```python
from build123d import *

# Parameters (mm, degrees)
SKETCH1_W               = 21.59
SKETCH1_H               = 46.99
BOSS_EXTRUDE1_DEPTH     = 76.2
SKETCH2_R               = 14.605
CUT_EXTRUDE1_DEPTH      = 93.090326311
CUT_EXTRUDE2_DEPTH      = 93.090326311
CUT_EXTRUDE3_REACH      = 94.09
SKETCH4_R               = 2.54
CUT_EXTRUDE4_REACH      = 94.09
CUT_EXTRUDE4_END_RADIUS = 14.605
SKETCH5_R               = 2.54
CHAMFER1_SIZE           = 2.54


with BuildPart() as part:
    # Sketch1 → Boss-Extrude1 (new body)
    with BuildSketch(Plane.XY):
        with Locations((10.795, 23.495)):
            Rectangle(SKETCH1_W, SKETCH1_H)
    extrude(amount=BOSS_EXTRUDE1_DEPTH)

    # Sketch2 → Cut-Extrude1 (cut, through all)
    with BuildSketch(Plane(origin=(21.59, 0, 0), x_dir=(0, 0, -1), z_dir=(1, 0, 0))):
        with Locations((-38.1, 23.495)):
            Circle(SKETCH2_R)
    extrude(amount=-CUT_EXTRUDE1_DEPTH, mode=Mode.SUBTRACT)

    # Sketch3 → Cut-Extrude2 (cut, through all)
    with BuildSketch(Plane(origin=(21.59, 0, 0), x_dir=(0, 0, -1), z_dir=(1, 0, 0))):
        Polygon((-50.8, 0), (-76.2, 23.495), (-76.2, 0), align=None)
    extrude(amount=-CUT_EXTRUDE2_DEPTH, mode=Mode.SUBTRACT)

    # Sketch4 → Cut-Extrude3 (cut, up to next)
    with BuildSketch(Plane(origin=(0, 46.99, 0), x_dir=(1, 0, 0), z_dir=(0, 1, 0)), mode=Mode.PRIVATE) as cut_extrude3_sk1:
        with Locations(Location((10.795, -12.7, 0), (0, 0, 270))):
            Circle(SKETCH4_R)
    cut_extrude3_tool1 = extrude(cut_extrude3_sk1.sketch, amount=-CUT_EXTRUDE3_REACH, mode=Mode.PRIVATE) & part.part
    # Sketch4 → Cut-Extrude3 (cut, up to next)
    with BuildSketch(Plane(origin=(0, 46.99, 0), x_dir=(1, 0, 0), z_dir=(0, 1, 0)), mode=Mode.PRIVATE) as cut_extrude3_sk2:
        with Locations(Location((10.795, -38.1, 0), (0, 0, 270))):
            Circle(SKETCH4_R)
    cut_extrude3_tool2 = extrude(cut_extrude3_sk2.sketch, amount=-CUT_EXTRUDE3_REACH, mode=Mode.PRIVATE) & part.part
    # Sketch4 → Cut-Extrude3 (cut, up to next)
    with BuildSketch(Plane(origin=(0, 46.99, 0), x_dir=(1, 0, 0), z_dir=(0, 1, 0)), mode=Mode.PRIVATE) as cut_extrude3_sk3:
        with Locations(Location((10.795, -63.5, 0), (0, 0, 270))):
            Circle(SKETCH4_R)
    cut_extrude3_tool3 = extrude(cut_extrude3_sk3.sketch, amount=-CUT_EXTRUDE3_REACH, mode=Mode.PRIVATE) & part.part
    add(cut_extrude3_tool1.solids().sort_by_distance((10.795, 46.99, 12.7))[0], mode=Mode.SUBTRACT)
    add(cut_extrude3_tool2.solids().sort_by_distance((10.795, 46.99, 38.1))[0], mode=Mode.SUBTRACT)
    add(cut_extrude3_tool3.solids().sort_by_distance((10.795, 46.99, 63.5))[0], mode=Mode.SUBTRACT)

    # Cut-Extrude4: up to this cylinder (the profile starts outside it)
    cut_extrude4_end = Plane(origin=(10.795, 23.495, 38.1), z_dir=(1, 0, 0)) * Cylinder(CUT_EXTRUDE4_END_RADIUS, 218.39, mode=Mode.PRIVATE)
    # Sketch5 → Cut-Extrude4 (cut, up to the surface)
    with BuildSketch(Plane.XZ, mode=Mode.PRIVATE) as cut_extrude4_sk1:
        with Locations(Location((10.795, 39.6875, 0), (0, 0, 270))):
            Circle(SKETCH5_R)
    cut_extrude4_tool1 = extrude(cut_extrude4_sk1.sketch, amount=-CUT_EXTRUDE4_REACH, mode=Mode.PRIVATE) - cut_extrude4_end
    add(cut_extrude4_tool1.solids().sort_by_distance((10.795, 0, 39.6875))[0], mode=Mode.SUBTRACT)

    # Chamfer1
    chamfer1_edges = [part.edges().sort_by_distance(p)[0] for p in [
        (0, 23.495, 52.705),
        (21.59, 23.495, 52.705),
        (21.59, 0, 25.4),
        (0, 0, 25.4),
        (0, 46.99, 38.1),
        (21.59, 46.99, 38.1),
    ]]
    chamfer(chamfer1_edges, length=CHAMFER1_SIZE)


solid = part.part
```
Here's how the part is built. I have some questions about the finished solid (model axes, mm). A direction names the side the tool comes from. Coordinates: 2 decimals unless noted, no trailing zeros. Loops run counter-clockwise (first coordinate to the right, second up) from the corner with the lowest first, then second, coordinate; pieces in that order, holes last. Notation, with made-up numbers: M 77.5,34.5 L 121.5,34.5 A17 cw 121.5,63.5 Z; hole C 63,74.5 d6. An arc over 180 degrees is marked long. One line per item, written item: value.
1. Please list where these lines run through material, in increasing order: probe 1 along Y at (x, z) = (15.25, 38.1); probe 2 along Z at (x, y) = (11.25, 34.5); probe 3 along Z at (x, y) = (3.25, 31).
Geometry says:
probe 1: y = 0 to 8.89, 38.1 to 46.99
probe 2: z = 0 to 10.2, 15.2 to 28.5, 47.7 to 61, 66 to 76.2
probe 3: z = 0 to 25.57, 50.63 to 76.2
2. Imagine slicing it at D-D (y = 5). List the corners of the cut face in (x, z) for me (1 decimal).
Geometry says:
outline: M 0,0 L 21.6,0 L 21.6,56.2 L 0,56.2 Z; hole C 10.8,12.7 d5.1; hole C 10.8,39.7 d5.1
3. Imagine slicing it at B-B (z = 38.1). List the corners of the cut face in (x, y) for me (3 decimals), and give its area (3 significant figures).
Geometry says:
outline: M 0,2.54 L 2.54,0 L 8.812,0 L 8.812,8.89 L 2.54,8.89 L 0,6.35 Z; M 0,40.64 L 2.54,38.1 L 8.255,38.1 L 8.255,46.99 L 2.54,46.99 L 0,44.45 Z; M 12.778,0 L 19.05,0 L 21.59,2.54 L 21.59,6.35 L 19.05,8.89 L 12.778,8.89 Z; M 13.335,38.1 L 19.05,38.1 L 21.59,40.64 L 21.59,44.45 L 19.05,46.99 L 13.335,46.99 Z
area: 278 mm2
4. Thinking about a two-plate mould opening in Z: for faces 3 (the flat face through (11, 0, 25)), 4 (the flat face through (11, 24, 0)), 5 (the cylindrical face through (10.907, 4.682, 42.225)), which applies, +Z half, -Z half, draft (parallel to the pull), parting line (faces both ways), or undercut?
Geometry says:
face 3: draft
face 4: -Z half
face 5: undercut
5. On a 3-axis mill with a long thin cutter (end or side, diameter ignored), from which of +Z, -Z, +X, -X, +Y, -Y can I reach the whole of each face in a straight line? I mean faces 1 (the cylindrical face through (10.907, 42.494, 35.562)), 2 (the flat face through (11, 35, 76.2)). Say none if no direction works.
Geometry says:
face 1: +Y
face 2: +Z, +X, -X, +Y, -Y
6. Imagine slicing it at A-A (z = 12.7). List the corners of the cut face in (x, y) for me (3 decimals).
Geometry says:
outline: M 0,2.54 L 2.54,0 L 8.255,0 L 8.255,46.99 L 2.54,46.99 L 0,44.45 Z; M 13.335,0 L 19.05,0 L 21.59,2.54 L 21.59,44.45 L 19.05,46.99 L 13.335,46.99 Z
7. Will these pins go through, and if not, where does the flat tip stop? pin 1 Ø1.5 at (y, z) = (39, 36) entering from +X; pin 2 Ø17.5 at (y, z) = (23.495, 38.1) entering from +X; pin 3 Ø1.5 at (x, y) = (3.5, 6) entering from +Z; pin 4 Ø4 at (x, z) = (10.8, 39.69) entering from -Y.
Geometry says:
pin 1: stops at x = 20.84
pin 2: passes through
pin 3: stops at z = 58.1
pin 4: stops at y = 37.65
8. Imagine slicing it at C-C (y = 21). State how many separate pieces and enclosed holes the cut face has, and give its area (3 significant figures).
Geometry says:
separate pieces: 2
enclosed holes: 2
area: 912 mm2
